Work out the finished part from the listing and answer in its coordinate system (mm). A direction names the side the tool comes from. Coordinates: 2 decimals unless noted, no trailing zeros.
1. Find the intervals of material crossed by probe 1 along X at (y, z) = (5, 1) (3 decimals); probe 2 along Z at (x, y) = (-364.5, 17.5) (3 decimals), in increasing order.
2. A tool of negligible diameter and unlimited length cuts with its end or side. For faces 1 (the flat face through (-356, -1, -3.175)), 2 (the flat face through (-609.6, -1, 0)), from which of +Z, -Z, +X, -X, +Y, -Y can it reach the whole face along a straight path? Write none if from no direction.
3. Determine the mould class of faces 3 (the flat face through (609.6, -1, 0)), 4 (the flat face through (-356, -1, 3.175)), 5 (the flat face through (355, -1, 3.175)), 6 (the flat face through (-9, 1, -12.7)) for opening direction Z: +Z half, -Z half, draft (parallel to the pull), parting line (faces both ways), or undercut.
```python
from build123d import *

# Parameters (mm, degrees)
F0_W     = 1219.2
F0_H     = 76.2
F1_DEPTH = 12.7
F2_W     = 31.75
F2_H     = 6.35
F3_DEPTH = 76.2
F4_DEPTH = 76.2


with BuildPart() as f1:
    # F0 (on Top) → F1 (new body, symmetric)
    with BuildSketch(Plane.XY):
        Rectangle(F0_W, F0_H)
    extrude(amount=F1_DEPTH, both=True)

    # F2 (on face) → F3 (cut, through all)
    with BuildSketch(Plane.XZ.offset(38.1)):
        with Locations((-355.6, 0)):
            Rectangle(F2_W, F2_H)
    extrude(amount=-F3_DEPTH, mode=Mode.SUBTRACT)

    # F2 (on face) → F4 (cut, through all)
    with BuildSketch(Plane.XZ.offset(38.1)):
        with Locations((355.6, 0)):
            Rectangle(F2_W, F2_H)
    extrude(amount=-F4_DEPTH, mode=Mode.SUBTRACT)


solid = f1.part
```
Geometry says:
1. probe 1: x = -609.6 to -371.475, -339.725 to 339.725, 371.475 to 609.6
1. probe 2: z = -12.7 to -3.175, 3.175 to 12.7
2. face 1: +Y, -Y
2. face 2: +Z, -Z, -X, +Y, -Y
3. face 3: draft
3. face 4: undercut
3. face 5: undercut
3. face 6: -Z half
